Geometry: final body of the model. Coordinates: model frame, mm. Coordinates: 2 decimals unless noted, no trailing zeros. Write each loop counter-clockwise with the first axis right and the second up, starting at its lowest first coordinate (ties: lowest second). Pieces come first, ordered by that corner, then holes.
from build123d import *

# Parameters (mm, degrees)
F0_R     = 1.765447
F1_DEPTH = 1
F3_DEPTH = 1


with BuildPart() as f1:
    # F0 (on Front) → F1 (new body, symmetric)
    with BuildSketch(Plane.XZ):
        with BuildLine():
            Line((5, -32.907251), (5, -8.660254))
            ThreePointArc((5, -8.660254), (0, 10), (-5, -8.660254))
            Line((-5, -8.660254), (-2.5, -17.104119))
            Line((-2.5, -17.104119), (-2.5, -22.222003))
            Line((-2.5, -22.222003), (0, -22.222003))
            Line((0, -22.222003), (-2.460267, -24.68227))
            Line((-2.460267, -24.68227), (0, -27.142537))
            Line((0, -27.142537), (-3.467242, -30.609779))
            Line((-3.467242, -30.609779), (0, -32.907251))
            Line((0, -32.907251), (-2.5, -32.907251))
            Line((-2.5, -32.907251), (-2.5, -34.345502))
            Line((-2.5, -34.345502), (0, -35.783753))
            Line((0, -35.783753), (5, -32.907251))
        make_face()
        with Locations((0, 6.308739)):
            Circle(F0_R, mode=Mode.SUBTRACT)
    extrude(amount=F1_DEPTH, both=True)

    # F2 (on face) → F3 (cut)
    with BuildSketch(Plane.XZ.offset(1)):
        with BuildLine():
            Line((3.160392, -32.907251), (3.160392, -8.660254))
            ThreePointArc((3.160392, -8.660254), (2.150394, -7.650256), (1.140397, -8.660254))
            Line((1.140397, -8.660254), (1.140397, -32.907251))
            ThreePointArc((1.140397, -32.907251), (2.150394, -33.917249), (3.160392, -32.907251))
        make_face()
    extrude(amount=-F3_DEPTH, mode=Mode.SUBTRACT)


solid = f1.part
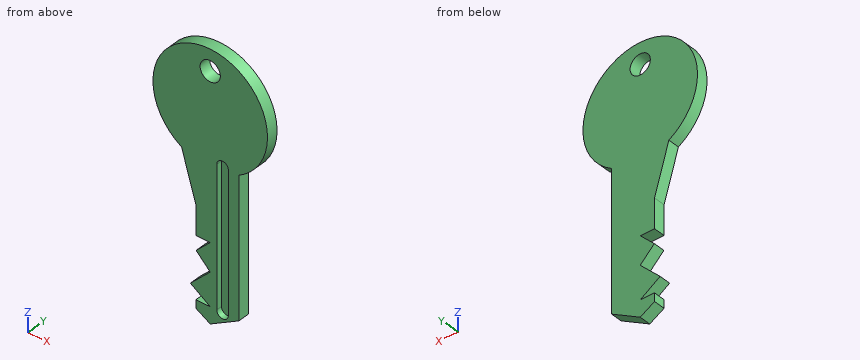
Item 1: Section B-B, the plane y = 0.55. Output: boundary loops of the cut face in (x, z), plus the area to 3 significant figures.
Derived:
outline: (-5, -8.66) - (-2.5, -17.1) - (-2.5, -22.22) - (0, -22.22) - (-2.46, -24.68) - (0, -27.14) - (-3.47, -30.61) - (0, -32.91) - (-2.5, -32.91) - (-2.5, -34.35) - (0, -35.78) - (5, -32.91) - (5, -8.66) arc R10 ccw (long way) to start; hole circle Ø3.53 at (0, 6.31)
area: 490 mm2
Item 2: Section C-C, the plane z = -12.5. Output: boundary loops of the cut face in (x, y).
Derived:
outline: (-3.86, -1) - (1.14, -1) - (1.14, 0) - (3.16, 0) - (3.16, -1) - (5, -1) - (5, 1) - (-3.86, 1) - close
Item 3: Pin query (flat end, axial travel): pin 1 (0.7 mm diameter, centred on y = 0.5, z = -33.5, fed in from -X); pin 2 (3 mm diameter, centred on x = 0, z = 6.31, fed in from -Y); pin 3 (0.8 mm diameter, centred on y = -0.5, z = -17, fed in from -X); pin 4 (1.6 mm diameter, centred on x = 2, z = -19.5, fed in from -Y). Return the tip coordinate at first contact, or that it passes through.
Derived:
pin 1: stops at x = -2.5
pin 2: passes through
pin 3: stops at x = -2.65
pin 4: stops at y = 0
Item 4: Section D-D, the plane x = -7.5. Output: boundary loops of the cut face in (y, z), plus the area to 3 significant figures.
Derived:
outline: (-1, -6.61) - (1, -6.61) - (1, 6.61) - (-1, 6.61) - close
area: 26.5 mm2
Item 5: Section A-A, the plane x = 0.5. Output: boundary loops of the cut face in (y, z).
Derived:
outline: (-1, -35.5) - (1, -35.5) - (1, 4.62) - (-1, 4.62) - close; (-1, 8) - (1, 8) - (1, 9.99) - (-1, 9.99) - close
Item 6: Material intervals for probe 1 along X at (y, z) = (-0.7, -20); probe 2 along X at (y, z) = (-0.9, -9); probe 3 along Z at (x, y) = (2.25, -0.1), sorted ascending.
Derived:
probe 1: x = -2.5 to 1.14, 3.16 to 5
probe 2: x = -4.9 to 1.14, 3.16 to 5
probe 3: z = -34.49 to -33.91, -7.66 to 9.74
